from build123d import *

# Parameters (mm, degrees)
F0_W     = 122.5
F0_H     = 122.5
F0_R     = 13.25
F1_DEPTH = 1
F2_DEPTH = 2
F3_R     = 2.55
F4_DEPTH = 2.001


# Not quite as in the source:
# - a feature names something its author has since deleted; it is built from what else it names


with BuildPart() as f1:
    # F0 (on Top) → F1 (new body)
    with BuildSketch(Plane.XY):
        Rectangle(F0_W, F0_H)
        with Locations((-45, -45)):
            Circle(F0_R, mode=Mode.SUBTRACT)
        with Locations((-15, -45)):
            Circle(F0_R, mode=Mode.SUBTRACT)
        with Locations((-45, -15)):
            Circle(F0_R, mode=Mode.SUBTRACT)
        with Locations((-15, -15)):
            Circle(F0_R, mode=Mode.SUBTRACT)
        with Locations((15, -45)):
            Circle(F0_R, mode=Mode.SUBTRACT)
        with Locations((45, -45)):
            Circle(F0_R, mode=Mode.SUBTRACT)
        with Locations((15, -15)):
            Circle(F0_R, mode=Mode.SUBTRACT)
        with Locations((45, -15)):
            Circle(F0_R, mode=Mode.SUBTRACT)
        with Locations((-45, 15)):
            Circle(F0_R, mode=Mode.SUBTRACT)
        with Locations((-15, 15)):
            Circle(F0_R, mode=Mode.SUBTRACT)
        with Locations((-45, 45)):
            Circle(F0_R, mode=Mode.SUBTRACT)
        with Locations((-15, 45)):
            Circle(F0_R, mode=Mode.SUBTRACT)
        with Locations((15, 15)):
            Circle(F0_R, mode=Mode.SUBTRACT)
        with Locations((45, 15)):
            Circle(F0_R, mode=Mode.SUBTRACT)
        with Locations((15, 45)):
            Circle(F0_R, mode=Mode.SUBTRACT)
        with Locations((45, 45)):
            Circle(F0_R, mode=Mode.SUBTRACT)
        with Locations((-45, 45)):
            Circle(F0_R)
        with Locations((-15, 45)):
            Circle(F0_R)
        with Locations((15, 45)):
            Circle(F0_R)
        with Locations((45, 45)):
            Circle(F0_R)
        with Locations((45, 15)):
            Circle(F0_R)
        with Locations((-15, 15)):
            Circle(F0_R)
        with Locations((-45, 15)):
            Circle(F0_R)
        with Locations((15, 15)):
            Circle(F0_R)
        with Locations((15, -15)):
            Circle(F0_R)
        with Locations((-15, -15)):
            Circle(F0_R)
        with Locations((-45, -15)):
            Circle(F0_R)
        with Locations((45, -15)):
            Circle(F0_R)
        with Locations((45, -45)):
            Circle(F0_R)
        with Locations((15, -45)):
            Circle(F0_R)
        with Locations((-15, -45)):
            Circle(F0_R)
        with Locations((-45, -45)):
            Circle(F0_R)
    extrude(amount=F1_DEPTH)

    # F0 (on Top) → F2 (join)
    with BuildSketch(Plane.XY):
        Rectangle(F0_W, F0_H)
        with Locations((-45, -45)):
            Circle(F0_R, mode=Mode.SUBTRACT)
        with Locations((-15, -45)):
            Circle(F0_R, mode=Mode.SUBTRACT)
        with Locations((-45, -15)):
            Circle(F0_R, mode=Mode.SUBTRACT)
        with Locations((-15, -15)):
            Circle(F0_R, mode=Mode.SUBTRACT)
        with Locations((15, -45)):
            Circle(F0_R, mode=Mode.SUBTRACT)
        with Locations((45, -45)):
            Circle(F0_R, mode=Mode.SUBTRACT)
        with Locations((15, -15)):
            Circle(F0_R, mode=Mode.SUBTRACT)
        with Locations((45, -15)):
            Circle(F0_R, mode=Mode.SUBTRACT)
        with Locations((-45, 15)):
            Circle(F0_R, mode=Mode.SUBTRACT)
        with Locations((-15, 15)):
            Circle(F0_R, mode=Mode.SUBTRACT)
        with Locations((-45, 45)):
            Circle(F0_R, mode=Mode.SUBTRACT)
        with Locations((-15, 45)):
            Circle(F0_R, mode=Mode.SUBTRACT)
        with Locations((15, 15)):
            Circle(F0_R, mode=Mode.SUBTRACT)
        with Locations((45, 15)):
            Circle(F0_R, mode=Mode.SUBTRACT)
        with Locations((15, 45)):
            Circle(F0_R, mode=Mode.SUBTRACT)
        with Locations((45, 45)):
            Circle(F0_R, mode=Mode.SUBTRACT)
    extrude(amount=F2_DEPTH)

    # F3 (on face) → F4 (cut, through all)
    with BuildSketch(Plane.XY.offset(2)):
        with Locations((-57.2, 57.2)):
            Circle(F3_R)
        with Locations((-30, 0)):
            Circle(F3_R)
        with Locations((57.2, 57.2)):
            Circle(F3_R)
        with Locations((30, 0)):
            Circle(F3_R)
        with Locations((57.2, -57.2)):
            Circle(F3_R)
        with Locations((-57.2, -57.2)):
            Circle(F3_R)
    extrude(amount=-F4_DEPTH, mode=Mode.SUBTRACT)


solid = f1.part
Build history of the part. All positions in model axes, mm. A direction names the side the tool comes from. Coordinates: 2 decimals unless noted, no trailing zeros. Order: outer loops, then holes, each group sorted by start corner. A loop starts at its lowest first (then second) coordinate and runs counter-clockwise, first axis right, second up. Notation, with made-up numbers: (-19.75, 62.25) - (33.25, 62.25) arc R25 ccw to (33.25, 82.25) - close; hole circle Ø5 at (-4.75, 63). An arc over 180 degrees is marked (long way). Write item = value, one per line. Start each with the question number.
1) Flat gauge pin, fed straight in: pin 1 Ø8 at (x, y) = (-39.5, 19) entering from +Z. Where does the tip first touch, or does it go through?
2) Saw through at D-D on y = 52. Write the cut outline in (x, z), then the cut area to 3 significant figures.
3) 3-axis set-ups, long thin cutter, end or side, ignore diameter. For faces 1 (the face through (52.123, 56.172, 1.493)), 2 (the face through (-56.02, -59.46, 1.01)): which of +Z, -Z, +X, -X, +Y, -Y reach the whole face in a straight line?
4) Saw through at B-B on z = 1.4. Count the separate pieces of the cut face and the enclosed holes in it, then the cut area to 3 significant figures.
5) Wall check: line 1 along X through (y, z) = (-45, 1.5); line 2 along Y through (x, z) = (14.5, 1.35); line 3 along Y through (x, z) = (-20.5, 1.55). Give the ranges that are in metal, low to high. Write a range as from..to.
6) Saw through at C-C on x = 45. Write the cut outline in (y, z).
7) Saw through at A-A on y = 0. Write the cut outline in (x, z).
From the geometry:
q1.pin_1 = 1
q2.outline = (-61.25, 0) - (61.25, 0) - (61.25, 2) - (56.25, 2) - (56.25, 1) - (33.75, 1) - (33.75, 2) - (26.25, 2) - (26.25, 1) - (3.75, 1) - (3.75, 2) - (-3.75, 2) - (-3.75, 1) - (-26.25, 1) - (-26.25, 2) - (-33.75, 2) - (-33.75, 1) - (-56.25, 1) - (-56.25, 2) - (-61.25, 2) - close
q2.area = 155 mm^2
q3.face_1 = +Z
q3.face_2 = +Z, -Z
q4.separate_pieces = 1
q4.enclosed_holes = 22
q4.area = 6,060 mm^2
q5.line_1 = -61.25..-58.25, -31.75..-28.25, -1.75..1.75, 28.25..31.75, 58.25..61.25
q5.line_2 = -61.25..-58.24, -31.76..-28.24, -1.76..1.76, 28.24..31.76, 58.24..61.25
q5.line_3 = -61.25..-57.05, -32.95..-27.05, -2.95..2.95, 27.05..32.95, 57.05..61.25
q6.outline = (-61.25, 0) - (61.25, 0) - (61.25, 2) - (58.25, 2) - (58.25, 1) - (31.75, 1) - (31.75, 2) - (28.25, 2) - (28.25, 1) - (1.75, 1) - (1.75, 2) - (-1.75, 2) - (-1.75, 1) - (-28.25, 1) - (-28.25, 2) - (-31.75, 2) - (-31.75, 1) - (-58.25, 1) - (-58.25, 2) - (-61.25, 2) - close
q7.outline = (-61.25, 0) - (-32.55, 0) - (-32.55, 2) - (-61.25, 2) - close; (-27.45, 0) - (27.45, 0) - (27.45, 2) - (-27.45, 2) - close; (32.55, 0) - (61.25, 0) - (61.25, 2) - (32.55, 2) - close
